Read the model definition and answer for the solid it produces. Units are mm, in the model's axes. Face numbers are marked on the shaded views. Coordinates: 2 decimals unless noted, no trailing zeros. Loops run counter-clockwise (first coordinate to the right, second up) from the corner with the lowest first, then second, coordinate; pieces in that order, holes last. Notation, with made-up numbers: (-37, 69) -> (13, 69) arc R14 cw to (13, 73) -> close; hole circle Ø7 at (-8.5, 33.5). An arc over 180 degrees is marked (long way). One line per question, with ' | ' between items. Start each with the question number.
```python
from build123d import *

# Parameters (mm, degrees)
ESQUISSE1_R                  = 32.5
BOSS_EXTRU_1_DEPTH           = 17
ESQUISSE2_R                  = 31
ENL_V_MAT_EXTRU_1_DEPTH      = 14
ESQUISSE3_W                  = 7
ESQUISSE3_H                  = 21.006684507
ENL_V_MAT_EXTRU_2_DEPTH      = 14
R_P_TITION_CIRCULAIRE1_COUNT = 2
R_P_TITION_CIRCULAIRE1_ANGLE = 70
D_GAGEMENT_M61_D             = 6.6
R_P_TITION_CIRCULAIRE2_COUNT = 3
R_P_TITION_CIRCULAIRE2_ANGLE = 160


with BuildPart() as part:
    # Esquisse1 → Boss.-Extru.1 (new body)
    with BuildSketch(Plane.XY):
        Circle(ESQUISSE1_R)
    extrude(amount=BOSS_EXTRU_1_DEPTH)

    # Esquisse2 → Enlèv. mat.-Extru.1 (cut)
    with BuildSketch(Plane.XY.offset(17)):
        Circle(ESQUISSE2_R)
    extrude(amount=-ENL_V_MAT_EXTRU_1_DEPTH, mode=Mode.SUBTRACT)

    # Esquisse3 → Enlèv. mat.-Extru.2 (cut)
    with BuildSketch(Plane.XY.offset(17)):
        with Locations((-2.367072337, 31.778784947)):
            Rectangle(ESQUISSE3_W, ESQUISSE3_H)
    enl_v_mat_extru_2 = extrude(amount=-ENL_V_MAT_EXTRU_2_DEPTH, mode=Mode.SUBTRACT)

    # Répétition circulaire1: Enlèv. mat.-Extru.2 ×2 about axis
    r_p_tition_circulaire1_axis = Axis((0, 0, 17), (0, 0, -1))
    for i in range(1, R_P_TITION_CIRCULAIRE1_COUNT):
        add(enl_v_mat_extru_2.rotate(r_p_tition_circulaire1_axis, i * R_P_TITION_CIRCULAIRE1_ANGLE / (R_P_TITION_CIRCULAIRE1_COUNT - 1)), mode=Mode.SUBTRACT)

    # Dégagement M61 (through all)
    with Locations(Plane.XY.offset(3)):
        with Locations((-14.965006824, 5.494015269)):
            d_gagement_m61 = Hole(D_GAGEMENT_M61_D / 2)

    # Répétition circulaire2: Dégagement M61 ×3 about axis
    r_p_tition_circulaire2_axis = Axis((0, 0, 0), (0, 0, 1))
    for i in range(1, R_P_TITION_CIRCULAIRE2_COUNT):
        add(d_gagement_m61.rotate(r_p_tition_circulaire2_axis, i * R_P_TITION_CIRCULAIRE2_ANGLE / (R_P_TITION_CIRCULAIRE2_COUNT - 1)), mode=Mode.SUBTRACT)


solid = part.part
```
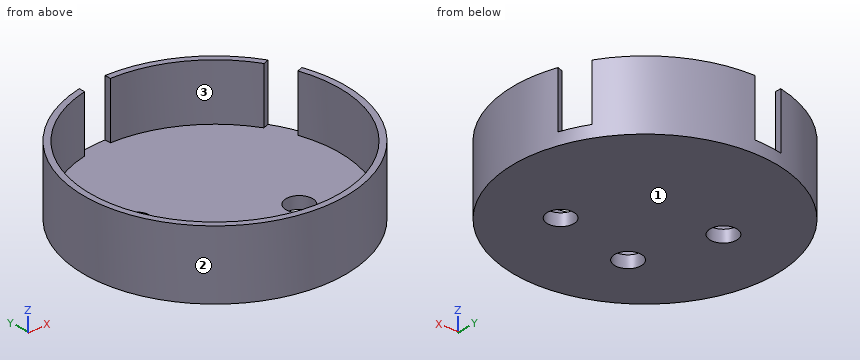
(1) Section B-B on x = -17.5 is taken. Write down the section's boundary in (y, z).
(2) Section A-A on z = 4.5 is taken. Write down the section's boundary in (x, y).
(3) Section C-C on y = 0 is taken. Write down the section's boundary in (x, z), plus the area to 3 significant figures.
(4) Section D-D on x = 0 is taken. Write down the section's boundary in (y, z), plus the area to 3 significant figures.
(5) Find the intervals of material crossed by probe 1 along X at (y, z) = (0, 13.75); probe 2 along Z at (x, y) = (11.5, -15.5); probe 3 along X at (y, z) = (18.5, 15), in increasing order. Write a range as from..to.
(6) Each of these flat-tipped pins is pushed along its axis until it touches: pin 1 Ø8 at (x, z) = (-17, 10) entering from +Y; pin 2 Ø6 at (x, y) = (-14.97, 5.49) entering from -Z; pin 3 Ø18.5 at (x, y) = (1, -2) entering from +Z; pin 4 Ø1.5 at (y, z) = (4, 10) entering from +X. Where does it stop, or does it pass through?
(7) Determine the mould class of the marked faces 1, 2 and 3 for opening direction Y: +Y half, -Y half, draft (parallel to the pull), parting line (faces both ways), or undercut.
Working result:
1) outline: (-27.39, 0) -> (3.38, 0) -> (3.38, 3) -> (-25.59, 3) -> (-25.59, 17) -> (-27.39, 17) -> close; (7.61, 0) -> (27.39, 0) -> (27.39, 17) -> (25.59, 17) -> (25.59, 3) -> (7.61, 3) -> close
2) outline: (-5.87, 30.44) -> (-5.87, 31.97) arc R32.5 ccw (long way) to (30.91, 10.04) -> (29.5, 9.53) arc R31 cw (long way) to start; (1.13, 30.98) arc R31 cw to (26.6, 15.92) -> (28.03, 16.45) arc R32.5 ccw to (1.13, 32.48) -> close
3) outline: (-32.5, 0) -> (32.5, 0) -> (32.5, 17) -> (31, 17) -> (31, 3) -> (-31, 3) -> (-31, 17) -> (-32.5, 17) -> close | area: 237 mm2
4) outline: (-32.5, 0) -> (32.5, 0) -> (32.5, 3) -> (-31, 3) -> (-31, 17) -> (-32.5, 17) -> close | area: 216 mm2
5) probe 1: x = -32.5..-31, 31..32.5 | probe 2: z = 0..3 | probe 3: x = -26.72..-24.87, 24.87..26.72
6) pin 1: stops at y = 29.79 | pin 2: passes through | pin 3: stops at z = 3 | pin 4: stops at x = 32.34
7) face 1: draft | face 2: parting line | face 3: undercut
